Autodesk Fusion 360 part; units mm, degrees
sketch "Sketch Metalens Holder" plane through (0, 0, 0) normal (1, 0, 0) x (0, 0, -1)
  line L0 (0, 8.15) -> (16.5, 8.15)
  line L1 (16.5, 8.15) -> (16.5, -8.35)
  line L2 (16.5, -8.35) -> (0, -8.35)
  line L3 (0, -8.35) -> (0, 8.15)
  dimension "d3" = 16.5
  dimension "d4" = 16.5
extrude "Extrude Metalens Holder" add sketch "Sketch Metalens Holder" along normal blind 12.95
shell "Shell Metalens Holder" thickness 1.1 removed faces 2 at (12.95, 2.65, -5.5) at (0, 2.65, -5.5)
sketch "Sketch Screwing Parts" plane through (0, 0, 0) normal (1, 0, 0) x (0, 0, -1)
  line L0 (4, 8.15) -> (4, 18.2)
  line L1 (4, 18.2) -> (11.49, 14.228)
  line L2 (11.49, 14.228) -> (9.515, 14.228)
  line L3 (9.515, 14.228) -> (9.515, 8.15)
  line L4 (4, 8.15) -> (9.515, 8.15)
  circle A0 centre (7, 13.4) radius 1.5
  line L5 (0, 8.15) -> (16.5, 8.15)
  line L6 (4.0564, -8.35) -> (4.0564, -18.4)
  line L7 (0.0564, -8.35) -> (16.5564, -8.35)
  line L8 (0, -8.35) -> (16.5, -8.35)
  line L9 (9.5564, -8.35) -> (9.5564, -14.428)
  line L10 (9.5564, -14.428) -> (11.5314, -14.428)
  line L11 (4.0564, -18.4) -> (11.5314, -14.428)
  circle A1 centre (7.0564, -13.6) radius 1.5
  point P0 (0, 8.15)
  dimension "d48" = 10.05
  dimension "d50" = 8.478
  dimension "d51" = 1.975
  dimension "d55" = 3
  dimension "d57" = 4.8
  dimension "d65" = 16.5
  dimension "d66" = 4
  dimension "d68" = 5.5
  dimension "d72" = 4.8
  dimension "d73" = 9.5
  dimension "d74" = 7
  dimension "d75" = 6.078
  dimension "d76" = 27
  dimension "d77" = 36.6
extrude "Extrude Crewing Parts" add sketch "Sketch Screwing Parts" along normal blind 12.95
ref_plane "WorkPlane1" through (9.95, -0.1, -8.25) normal (1, 0, 0) x (0, 0, -1)
sketch "Sketch Inside Slit" plane through (9.95, 0, 0) normal (1, 0, 0) x (0, 0, -1)
  line L0 (15.4, 7.05) -> (15.4, -7.25)
  line L1 (0.5, 7.65) -> (16, 7.65)
  line L2 (16, 7.65) -> (16, -7.85)
  line L3 (16, -7.85) -> (0.5, -7.85)
  line L4 (0.5, -7.85) -> (0.5, 7.65)
  line L5 (15.4, 7.05) -> (1.1, 7.05)
  line L6 (1.1, 7.05) -> (1.1, -7.25)
  line L7 (1.1, -7.25) -> (15.4, -7.25)
  line L8 (15.4, -7.25) -> (15.4, 7.05)
  line L9 (15.4, 7.05) -> (0.5, 7.05)
  line L10 (1.1, 7.05) -> (16, 7.05)
  line L11 (1.1, -7.25) -> (16, -7.25)
  line L12 (15.4, -7.25) -> (0.5, -7.25)
  line L13 (16.5, -8.35) -> (16.5, 8.15)
  line L14 (16.5, 8.15) -> (9.515, 8.15)
  point P0 (1.1, -7.25)
  point P1 (1.1, 7.05)
  dimension "d91" = 15.5
  dimension "d132" = 0.5
  dimension "d133" = 0.5
extrude "Extrude Inside Slit" cut sketch "Sketch Inside Slit" along normal mid plane 0.8
extrude "Extrude Remove 4th Wall" cut 2 faces at (3.1833, 2.2833, -15.4) (11.2167, 2.2833, -15.4) along direction (0, 0, -1) blind 1.1
extrude "Extrude Remove 4th Wall Bis" cut 1 faces at (10.0833, -2.4833, -16) along direction (0, 0, -1) blind 0.6
Geometry: final body of the model. Coordinates: model frame, mm. A direction names the side the tool comes from. Coordinates: 2 decimals unless noted, no trailing zeros. Order: outer loops, then holes, each group sorted by start corner. A loop starts at its lowest first (then second) coordinate and runs counter-clockwise, first axis right, second up. Notation, with made-up numbers: (28, -40) - (42, -40) arc R34 ccw to (42, -8) - close; hole circle Ø6 at (-4, 31.25). An arc over 180 degrees is marked (long way). Return JSON: item names as keys, results as strings. Group by question number.
1. Pin query (flat end, axial travel): pin 1 (5 mm diameter, centred on x = 3, z = -7.5, fed in from -Y); pin 2 (0.9 mm diameter, centred on x = 10, z = -5.5, fed in from +Y); pin 3 (1.6 mm diameter, centred on x = 8, z = -10.5, fed in from -Y); pin 4 (1.5 mm diameter, centred on x = 2, y = -8.5, fed in from +Z). Return the tip coordinate at first contact, or that it passes through.
2. Cut plane A-A (y = 13.4). Output: boundary loops of the cut face in (x, z) (3 decimals).
3. Cut plane C-C (x = 5). Output: boundary loops of the cut face in (y, z) (3 decimals), plus the area to 3 significant figures.
4. Material intervals for line 1 along Y through (x, z) = (3.75, -1.5); line 2 along Y through (x, z) = (3.25, -7); line 3 along Z through (x, y) = (1.5, -12), sorted ascending. Write a range as [from, to].
5. Cut plane D-D (y = -5). Output: boundary loops of the cut face in (x, z), plus the area to 3 significant figures.
6. Cut plane B-B (z = -14). Output: boundary loops of the cut face in (x, y).
7. Pull-direction query (X, two-part tool) for faces 1 (the face through (12.95, -1.4, -0.9)), 2 (the face through (0, -1.4, -0.9)), 3 (the face through (10.35, -0.1, -0.8)), 4 (the face through (6, -14.428, -11)); classes: pulls with the +X half, pulls with the -X half, needs draft (parallel to the pull), parting line crosses it, or undercut.
8. Set-up query: faces 5 (the face through (12, 0, -1.1)), 6 (the face through (6.38, 12.39, -5.89)), 7 (the face through (6, -13, -4.056)), 8 (the face through (6, 13, -4)), 9 (the face through (6, 0, 0)). Return all of +Z, -Z, +X, -X, +Y, -Y with unobstructed straight access to the full face (end or side cutting, diameter ignored); none if empty.
Resolved:
{
 "1": {"pin 1": "stops at y = -17.9", "pin 2": "stops at y = 17.64", "pin 3": "stops at y = -15.4", "pin 4": "stops at z = 0"},
 "2": {"outline": "(0, -9.515) - (12.95, -9.515) - (12.95, -8.5) - (0, -8.5) - close; (0, -5.5) - (12.95, -5.5) - (12.95, -4) - (0, -4) - close"},
 "3": {"outline": "(-18.4, -4.056) - (-14.428, -11.531) - (-14.428, -9.556) - (-8.35, -9.556) - (-8.35, -16.5) - (-7.25, -16.5) - (-7.25, -1.1) - (7.05, -1.1) - (7.05, -16.5) - (8.15, -16.5) - (8.15, -9.515) - (14.228, -9.515) - (14.228, -11.49) - (18.2, -4) - (8.15, -4) - (8.15, 0) - (-8.35, 0) - (-8.35, -4.056) - close; hole circle Ø3 at (-13.6, -7.056); hole circle Ø3 at (13.4, -7)", "area": "135 mm²"},
 "4": {"line 1": "y = [-8.35, -7.25], [7.05, 8.15]", "line 2": "y = [-16.84, -15.1], [-12.1, -7.25], [7.05, 11.9], [14.9, 16.61]", "line 3": "z = [-9.56, -4.06]"},
 "5": {"outline": "(0, -1.1) - (9.55, -1.1) - (9.55, -0.5) - (10.35, -0.5) - (10.35, -1.1) - (12.95, -1.1) - (12.95, 0) - (0, 0) - close", "area": "13.8 mm²"},
 "6": {"outline": "(0, -8.35) - (12.95, -8.35) - (12.95, -7.25) - (10.35, -7.25) - (10.35, -7.85) - (9.55, -7.85) - (9.55, -7.25) - (0, -7.25) - close; (0, 7.05) - (9.55, 7.05) - (9.55, 7.65) - (10.35, 7.65) - (10.35, 7.05) - (12.95, 7.05) - (12.95, 8.15) - (0, 8.15) - close"},
 "7": {"face 1": "pulls with the +X half", "face 2": "pulls with the -X half", "face 3": "undercut", "face 4": "needs draft"},
 "8": {"face 5": "-Z, +X, -X", "face 6": "+X, -X", "face 7": "+Z, +X, -X, -Y", "face 8": "+Z, +X, -X, +Y", "face 9": "+Z, +X, -X, +Y, -Y"}
}
